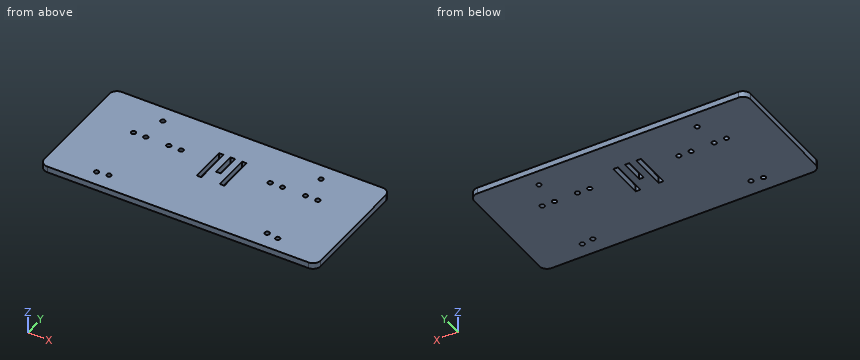
```python
from build123d import *

# Parameters (mm, degrees)
SKETCH1_W           = 180
SKETCH1_H           = 80
SKETCH1_R           = 1.5
BOSS_EXTRUDE1_DEPTH = 4
SKETCH2_W           = 3
SKETCH2_H           = 24
SKETCH2_H_2         = 15.4
CUT_EXTRUDE1_DEPTH  = 4
FILLET1_R           = 5


with BuildPart() as part:
    # Sketch1 → Boss-Extrude1 (new body)
    with BuildSketch(Plane.XY):
        with Locations((2.700642055, -21.117125984)):
            Rectangle(SKETCH1_W, SKETCH1_H)
        with Locations((-57.299357945, -9.617125984)):
            Circle(SKETCH1_R, mode=Mode.SUBTRACT)
        with Locations((62.700642055, -9.617125984)):
            Circle(SKETCH1_R, mode=Mode.SUBTRACT)
        with Locations((61.700642055, -51.117125984)):
            Circle(SKETCH1_R, mode=Mode.SUBTRACT)
        with Locations((-56.299357945, -51.117125984)):
            Circle(SKETCH1_R, mode=Mode.SUBTRACT)
        with Locations((-49.299357945, -9.617125984)):
            Circle(SKETCH1_R, mode=Mode.SUBTRACT)
        with Locations((54.700642055, -9.617125984)):
            Circle(SKETCH1_R, mode=Mode.SUBTRACT)
        with Locations((-34.299357945, -9.617125984)):
            Circle(SKETCH1_R, mode=Mode.SUBTRACT)
        with Locations((-26.299357945, -9.617125984)):
            Circle(SKETCH1_R, mode=Mode.SUBTRACT)
        with Locations((39.700642055, -9.617125984)):
            Circle(SKETCH1_R, mode=Mode.SUBTRACT)
        with Locations((31.700642055, -9.617125984)):
            Circle(SKETCH1_R, mode=Mode.SUBTRACT)
        with Locations((-48.799357945, 7.882874016)):
            Circle(SKETCH1_R, mode=Mode.SUBTRACT)
        with Locations((54.200642055, 7.882874016)):
            Circle(SKETCH1_R, mode=Mode.SUBTRACT)
        with Locations((54.200642055, -50.117125984)):
            Circle(SKETCH1_R, mode=Mode.SUBTRACT)
        with Locations((-48.799357945, -50.117125984)):
            Circle(SKETCH1_R, mode=Mode.SUBTRACT)
    extrude(amount=BOSS_EXTRUDE1_DEPTH)

    # Sketch2 → Cut-Extrude1 (cut)
    with BuildSketch(Plane.XY.offset(4)):
        with Locations((-5.299357945, -13.117125984)):
            Rectangle(SKETCH2_W, SKETCH2_H)
        with Locations((2.200642055, -8.817125984)):
            Rectangle(SKETCH2_W, SKETCH2_H_2)
        with Locations((9.700642055, -13.117125984)):
            Rectangle(SKETCH2_W, SKETCH2_H)
    extrude(amount=-CUT_EXTRUDE1_DEPTH, mode=Mode.SUBTRACT)

    # Fillet1
    fillet1_edges = [part.edges().sort_by_distance(p)[0] for p in [
        (-87.299357945, 18.882874016, 2),
        (92.700642055, 18.882874016, 2),
        (92.700642055, -61.117125984, 2),
        (-87.299357945, -61.117125984, 2),
    ]]
    fillet(fillet1_edges, radius=FILLET1_R)


solid = part.part
```
Geometry check sheet. Reference: the model listing, model coordinates, mm. Coordinates: 2 decimals unless noted, no trailing zeros. Order: outer loops, then holes, each group sorted by start corner. A loop starts at its lowest first (then second) coordinate and runs counter-clockwise, first axis right, second up. Notation, with made-up numbers: (-38.5, -5) - (15.5, -5) arc R12 ccw to (15.5, 1) - close; hole circle Ø2 at (40.5, 13.5). An arc over 180 degrees is marked (long way). Use one line per item in the form item = value.
1. Section check B-B (z = 0.9). State how many separate pieces and enclosed holes the cut face has, then the cut area to 3 significant figures.
Here are the results:
separate_pieces = 1
enclosed_holes = 17
area = 14,100 mm²
2. Scan lines: line 1 (X direction, y = -15, z = 1.75); line 2 (Y direction, x = -56.5, z = 0.6); line 3 (Y direction, x = 31.5, z = 3.6). Record each from-to range of solid material in increasing order.
Here are the results:
line_1 = -87.3 to -6.8, -3.8 to 0.7, 3.7 to 8.2, 11.2 to 92.7
line_2 = -61.12 to -52.6, -49.63 to -10.89, -8.35 to 18.88
line_3 = -61.12 to -11.1, -8.13 to 18.88
3. Section check A-A (y = -13). Record the boundary of the cut face in (x, z), then the cut area to 3 significant figures.
Here are the results:
outline = (-87.3, 0) - (-6.8, 0) - (-6.8, 4) - (-87.3, 4) - close; (-3.8, 0) - (0.7, 0) - (0.7, 4) - (-3.8, 4) - close; (3.7, 0) - (8.2, 0) - (8.2, 4) - (3.7, 4) - close; (11.2, 0) - (92.7, 0) - (92.7, 4) - (11.2, 4) - close
area = 684 mm²
4. Gauge pin test, flat end, axial feed: pin 1 (2.5 mm diameter, centred on x = -57.3, y = -9.62, fed in from -Z). Record the tip position at first contact, or that the pin passes through.
Here are the results:
pin_1 = through
